Read the model definition and answer for the solid it produces. Units are mm, in the model's axes. Coordinates: 2 decimals unless noted, no trailing zeros. Order: outer loops, then holes, each group sorted by start corner. A loop starts at its lowest first (then second) coordinate and runs counter-clockwise, first axis right, second up. Notation, with made-up numbers: M 74,34 L 111,34 A37 ccw 111,70 Z; hole C -1.75,41.5 d4. An arc over 180 degrees is marked long. Use a Markdown table: item, result. Add a question column.
1) Find section B-B on y = -4. Count the separate pieces of the cut face and the enclosed holes in it, plus the area to 3 significant figures.
2) Each of these flat-tipped pins is pushed along its axis until it touches: pin 1 Ø1 at (y, z) = (2, 3) entering from -X; pin 2 Ø20 at (x, y) = (-47.53, 2.82) entering from -Z; pin 3 Ø5 at (x, y) = (-49.5, -18) entering from +Z. Where does it stop, or does it pass through?
3) Find section A-A on z = 4.5. Write down the section's boundary in (x, y).
4) The mould has two halves that part along Y. Classify faces 1 (the face through (45.314, 8.727, 6.174)), 2 (the face through (-6.088, 14.483, 6.174)), 3 (the face through (23, -2, 7)): released by +Y, released by -Y, zero draft, split by the parting line, or undercut.
5) Find the intervals of material crossed by probe 1 along X at (y, z) = (4, 3.5) (3 decimals); probe 2 along X at (y, z) = (-4.5, 3.75); probe 3 along X at (y, z) = (27, 1), in increasing order. Write a range as [from, to].
from build123d import *

# Parameters (mm, degrees)
F1_DEPTH     = 7
F2_T2_ANGLE  = 57.1143931605
F2_T4_ANGLE  = 57.1143931605
F2_T6_ANGLE  = 76.6293726343
F2_T8_ANGLE  = 76.6293726343
F2_T10_ANGLE = 57.1143931605
F2_T12_ANGLE = 76.6293726343
F2_T14_ANGLE = 76.6293726343
F2_T16_ANGLE = 57.1143931605


# Not quite as in the source:
# - a fillet or chamfer that OpenCascade refuses, or shapes differently, is made with other operations: its cross-section is extruded or revolved along the edge and cut away or added


with BuildPart() as f1:
    # F0 (on Top) → F1 (new body)
    with BuildSketch(Plane.XY):
        with BuildLine():
            ThreePointArc((-51.9588312409, 22.6017753357), (-59.8237606638, 25.7612832302), (-67.4684691244, 29.4216162089))
            ThreePointArc((-67.4684691244, 29.4216162089), (-61.2035945552, 16.7707381256), (-59.0483218899, 2.8191013262))
            Line((-59.0483218899, 2.8191013262), (-58.7843277942, 2.8191013262))
            ThreePointArc((-58.7843277942, 2.8191013262), (-47.5343277942, 14.0691013262), (-36.2843277942, 2.8191013262))
            Line((-36.2843277942, 2.8191013262), (-18.2192023098, 2.8191013262))
            ThreePointArc((-18.2192023098, 2.8191013262), (-17.978724805, 5.1327379505), (-17.267573078, 7.3474630081))
            Line((-17.267573078, 7.3474630081), (-51.9588312409, 22.6017753357))
        make_face()
        with BuildLine():
            ThreePointArc((-6.9692023098, 14.6539675384), (-29.8123323501, 16.6561845448), (-51.9588312409, 22.6017753357))
            Line((-51.9588312409, 22.6017753357), (-17.267573078, 7.3474630081))
            ThreePointArc((-17.267573078, 7.3474630081), (-13.1181221775, 12.2399974863), (-6.9692023098, 14.0691013262))
            Line((-6.9692023098, 14.0691013262), (-6.9692023098, 14.6539675384))
        make_face()
        with BuildLine():
            Line((-58.7843277942, 2.8191013262), (-59.0483218899, 2.8191013262))
            ThreePointArc((-59.0483218899, 2.8191013262), (-61.2035945552, -11.1325354733), (-67.4684691244, -23.7834135565))
            ThreePointArc((-67.4684691244, -23.7834135565), (-38.1069797367, -12.7610910953), (-6.9692023098, -9.0157648861))
            Line((-6.9692023098, -9.0157648861), (-6.9692023098, -8.4308986738))
            ThreePointArc((-6.9692023098, -8.4308986738), (-14.9241535982, -5.1358499622), (-18.2192023098, 2.8191013262))
            Line((-18.2192023098, 2.8191013262), (-36.2843277942, 2.8191013262))
            ThreePointArc((-36.2843277942, 2.8191013262), (-47.5343277942, -8.4308986738), (-58.7843277942, 2.8191013262))
        make_face()
        with BuildLine():
            ThreePointArc((45.1099172702, 2.8191013262), (47.2651899355, 16.7707381256), (53.5300645047, 29.4216162089))
            ThreePointArc((53.5300645047, 29.4216162089), (24.168575117, 18.3992937476), (-6.9692023098, 14.6539675384))
            Line((-6.9692023098, 14.6539675384), (-6.9692023098, 14.0691013262))
            ThreePointArc((-6.9692023098, 14.0691013262), (0.9857489785, 10.7740526145), (4.2807976902, 2.8191013262))
            Line((4.2807976902, 2.8191013262), (22.3459231745, 2.8191013262))
            ThreePointArc((22.3459231745, 2.8191013262), (33.5959231745, 14.0691013262), (44.8459231745, 2.8191013262))
            Line((44.8459231745, 2.8191013262), (45.1099172702, 2.8191013262))
        make_face()
        with BuildLine():
            ThreePointArc((53.5300645047, -23.7834135565), (47.2651899355, -11.1325354733), (45.1099172702, 2.8191013262))
            Line((45.1099172702, 2.8191013262), (44.8459231745, 2.8191013262))
            ThreePointArc((44.8459231745, 2.8191013262), (33.5959231745, -8.4308986738), (22.3459231745, 2.8191013262))
            Line((22.3459231745, 2.8191013262), (4.2807976902, 2.8191013262))
            ThreePointArc((4.2807976902, 2.8191013262), (4.0403201853, 0.5054647019), (3.3291684583, -1.7092603557))
            Line((3.3291684583, -1.7092603557), (38.0204266212, -16.9635726834))
            ThreePointArc((38.0204266212, -16.9635726834), (45.8853560441, -20.1230805779), (53.5300645047, -23.7834135565))
        make_face()
        with BuildLine():
            Line((-6.9692023098, -8.4308986738), (-6.9692023098, -9.0157648861))
            ThreePointArc((-6.9692023098, -9.0157648861), (15.8739277304, -11.0179818925), (38.0204266212, -16.9635726834))
            Line((38.0204266212, -16.9635726834), (3.3291684583, -1.7092603557))
            ThreePointArc((3.3291684583, -1.7092603557), (-0.8202824422, -6.601794834), (-6.9692023098, -8.4308986738))
        make_face()
    extrude(amount=F1_DEPTH)

    # F2: chamfer of 1 on 8 edges, made by hand

    # F2_s1 → F2_t2 (revolve, cut)
    with BuildSketch(Plane(origin=(-64.2958342843, -34.9929409524, 0), x_dir=(0, 0, 1), z_dir=(-0.8783403422, -0.4780358179, 0))):
        Polygon((6, 11.3876031391), (7, 12.3876031391), (7, 11.3876031391), align=None)
    revolve(axis=Axis((-6.9692023098, -140.3245743959, 7), (0, 0, -1)), revolution_arc=F2_T2_ANGLE, mode=Mode.SUBTRACT)

    # F2_s3 → F2_t4 (revolve, cut)
    with BuildSketch(Plane(origin=(55.9099674663, 30.4289416566, 0), x_dir=(0, 0, 1), z_dir=(0.8783403422, 0.4780358179, 0))):
        Polygon((6, -0.2277143611), (7, 0.7722856389), (7, -0.2277143611), align=None)
    revolve(axis=Axis((-6.9692023098, 145.9627770483, 7), (0, 0, -1)), revolution_arc=F2_T4_ANGLE, mode=Mode.SUBTRACT)

    # F2_s5 → F2_t6 (revolve, cut)
    with BuildSketch(Plane(origin=(-41.8392456248, 52.9497637497, 0), x_dir=(0, 0, 1), z_dir=(-0.6199801689, 0.7846174801, 0))):
        Polygon((6, -34.6245823345), (7, -33.6245823345), (7, -34.6245823345), align=None)
    revolve(axis=Axis((-105.2822329994, 2.8191013262, 7), (0, 0, -1)), revolution_arc=F2_T6_ANGLE, mode=Mode.SUBTRACT)

    # F2_s7 → F2_t8 (revolve, cut)
    with BuildSketch(Plane(origin=(-41.8392456248, 52.9497637497, 0), x_dir=(0, 0, 1), z_dir=(-0.6199801689, 0.7846174801, 0))):
        Polygon((1, -34.6245823345), (0, -33.6245823345), (0, -34.6245823345), align=None)
    revolve(axis=Axis((-105.2822329994, 2.8191013262, 0), (0, 0, -1)), revolution_arc=F2_T8_ANGLE, mode=Mode.SUBTRACT)

    # F2_s9 → F2_t10 (revolve, cut)
    with BuildSketch(Plane(origin=(55.9099674663, 30.4289416566, 0), x_dir=(0, 0, 1), z_dir=(0.8783403422, 0.4780358179, 0))):
        Polygon((1, -0.2277143611), (0, 0.7722856389), (0, -0.2277143611), align=None)
    revolve(axis=Axis((-6.9692023098, 145.9627770483, 0), (0, 0, -1)), revolution_arc=F2_T10_ANGLE, mode=Mode.SUBTRACT)

    # F2_s11 → F2_t12 (revolve, cut)
    with BuildSketch(Plane(origin=(33.7389773041, -42.6984485674, 0), x_dir=(0, 0, 1), z_dir=(0.6199801689, -0.7846174801, 0))):
        Polygon((1, -27.1838402573), (0, -26.1838402573), (0, -27.1838402573), align=None)
    revolve(axis=Axis((91.3438283797, 2.8191013262, 0), (0, 0, -1)), revolution_arc=F2_T12_ANGLE, mode=Mode.SUBTRACT)

    # F2_s13 → F2_t14 (revolve, cut)
    with BuildSketch(Plane(origin=(33.7389773041, -42.6984485674, 0), x_dir=(0, 0, 1), z_dir=(0.6199801689, -0.7846174801, 0))):
        Polygon((6, -27.1838402573), (7, -26.1838402573), (7, -27.1838402573), align=None)
    revolve(axis=Axis((91.3438283797, 2.8191013262, 7), (0, 0, -1)), revolution_arc=F2_T14_ANGLE, mode=Mode.SUBTRACT)

    # F2_s15 → F2_t16 (revolve, cut)
    with BuildSketch(Plane(origin=(-64.2958342843, -34.9929409524, 0), x_dir=(0, 0, 1), z_dir=(-0.8783403422, -0.4780358179, 0))):
        Polygon((1, 11.3876031391), (0, 12.3876031391), (0, 11.3876031391), align=None)
    revolve(axis=Axis((-6.9692023098, -140.3245743959, 0), (0, 0, -1)), revolution_arc=F2_T16_ANGLE, mode=Mode.SUBTRACT)


solid = f1.part
Check result:
| question | item | result |
|---|---|---|
| 1 | separate pieces | 4 |
| 1 | enclosed holes | 0 |
| 1 | area | 358 mm2 |
| 2 | pin 1 | stops at x = -59.07 |
| 2 | pin 2 | passes through |
| 2 | pin 3 | stops at z = 6.7 |
| 3 | outline | M -67.47,-23.78 A131.31 cw 53.53,-23.78 A46.23 cw 53.53,29.42 A131.31 cw -67.47,29.42 A46.23 cw Z; hole C -47.53,2.82 d22.5; hole C -6.97,2.82 d22.5; hole C 33.6,2.82 d22.5 |
| 4 | face 1 | undercut |
| 4 | face 2 | released by +Y |
| 4 | face 3 | zero draft |
| 5 | probe 1 | x = [-59.063, -58.722], [-36.346, -18.157], [4.219, 22.408], [44.784, 45.125] |
| 5 | probe 2 | x = [-59.63, -56.08], [-38.99, -15.51], [1.57, 25.05], [42.14, 45.69] |
| 5 | probe 3 | x = [-65.88, -62.56], [48.62, 51.94] |
